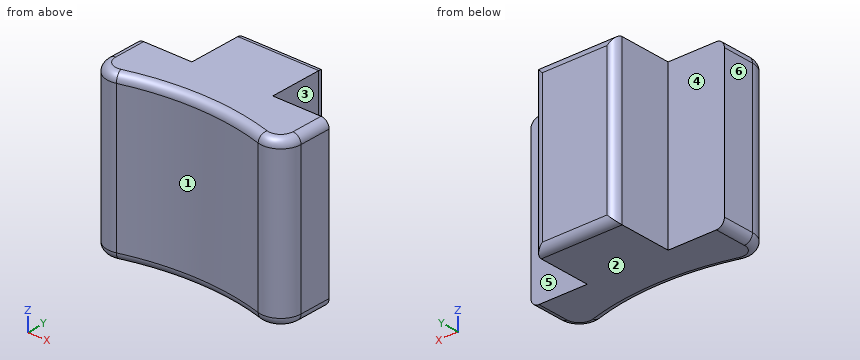
from build123d import *

# Parameters (mm, degrees)
BOSS_EXTRUDE1_DEPTH = 50.8
FILLET1_R           = 6.35
FILLET3_R           = 2.54
FILLET4_R           = 2.54
FILLET5_R           = 2.54


with BuildPart() as part:
    # Sketch1 → Boss-Extrude1 (new body)
    with BuildSketch(Plane.XY):
        with BuildLine():
            Line((-12.7, 111.432937893), (12.7, 111.432937893))
            Line((12.7, 111.432937893), (12.7, 92.382937893))
            Line((12.7, 92.382937893), (30.375497444, 92.382937893))
            Line((30.375497444, 92.382937893), (30.375497444, 73.332937893))
            ThreePointArc((30.375497444, 73.332937893), (0, 79.375), (-30.375497444, 73.332937893))
            Line((-30.375497444, 73.332937893), (-30.375497444, 92.382937893))
            Line((-30.375497444, 92.382937893), (-12.7, 92.382937893))
            Line((-12.7, 92.382937893), (-12.7, 111.432937893))
        make_face()
    extrude(amount=BOSS_EXTRUDE1_DEPTH)

    # Fillet1
    fillet1_edges = [part.edges().sort_by_distance(p)[0] for p in [
        (30.375497444, 73.332937893, 25.4),
        (-30.375497444, 73.332937893, 25.4),
    ]]
    fillet(fillet1_edges, radius=FILLET1_R)

    # Fillet3
    fillet3_edges = [part.edges().sort_by_distance(p)[0] for p in [
        (-12.7, 111.432937893, 25.4),
        (12.7, 111.432937893, 25.4),
        (0, 111.432937893, 50.8),
        (0, 111.432937893, 0),
    ]]
    fillet(fillet3_edges, radius=FILLET3_R)

    # Fillet4
    fillet4_edges = [part.edges().sort_by_distance(p)[0] for p in [
        (0, 79.375, 50.8),
        (30.375497444, 87.336186401, 50.8),
        (27.834803015, 77.208914161, 50.8),
        (-27.834803015, 77.208914161, 50.8),
        (-30.375497444, 87.336186401, 50.8),
    ]]
    fillet(fillet4_edges, radius=FILLET4_R)

    # Fillet5
    fillet5_edges = [part.edges().sort_by_distance(p)[0] for p in [
        (-30.375497444, 87.336186401, 0),
        (0, 79.375, 0),
        (30.375497444, 87.336186401, 0),
        (27.834803015, 77.208914161, 0),
        (-27.834803015, 77.208914161, 0),
    ]]
    fillet(fillet5_edges, radius=FILLET5_R)


solid = part.part
Work out the finished part from the listing and answer in its coordinate system (mm). Face numbers are marked on the shaded views. A direction names the side the tool comes from. Coordinates: 2 decimals unless noted, no trailing zeros. Loops run counter-clockwise (first coordinate to the right, second up) from the corner with the lowest first, then second, coordinate; pieces in that order, holes last. Notation, with made-up numbers: M -35,38.25 L -13,38.25 A22 ccw -13,75.25 Z; hole C -12,25 d1. An arc over 180 degrees is marked long. Answer in a Markdown table with one row per item. Add a question column.
1. Flat-ended cylindrical pins translate along their axes: P1, Ø12, axis at x = 4.5, y = 101.5, coming from the -Z side; P2, Ø2, axis at y = 106.5, z = 33.5, coming from the +X side; P3, Ø5.5, axis at x = 23.5, z = 19.5, coming from the +Y side; P4, Ø5, axis at y = 99, z = 13.5, coming from the -X side. Find the tip coordinate at first contact, or state that the pin passes through.
2. Find section B-B, the plane x = 0. Write down the section's boundary in (y, z) (3 decimals), then the cut area to 3 significant figures.
3. A tool of negligible diameter and unlimited length cuts with its end or side. For the marked faces 4, 5 and 6, from which of +Z, -Z, +X, -X, +Y, -Y can it reach the whole face along a straight path? Write none if from no direction.
4. The mould has two halves that part along X. Classify the marked faces 1, 2 and 3: pulls with the +X half, pulls with the -X half, needs draft (parallel to the pull), parting line crosses it, or undercut.
5. Consider L1, parallel to X at y = 108, z = 38; L2, parallel to X at y = 85, z = 48.5; L3, parallel to Y at x = -24, z = 44. Determine where each line is inside the solid, lowest interval first.
6. Find section C-C, the plane y = 101. Write down the section's boundary in (x, z), then the cut area to 3 significant figures.
Reported:
| question | item | result |
|---|---|---|
| 1 | P1 | stops at z = 0 |
| 1 | P2 | stops at x = 12.7 |
| 1 | P3 | stops at y = 92.38 |
| 1 | P4 | stops at x = -12.7 |
| 2 | outline | M 79.375,2.54 A2.54 ccw 81.915,0 L 108.893,0 A2.54 ccw 111.433,2.54 L 111.433,48.26 A2.54 ccw 108.893,50.8 L 81.915,50.8 A2.54 ccw 79.375,48.26 Z |
| 2 | area | 1,620 mm^2 |
| 3 | face 4 | +Z, -Z, -X, +Y |
| 3 | face 5 | +Z, -Z, +X, +Y |
| 3 | face 6 | +Z, -Z, -X, +Y, -Y |
| 4 | face 1 | undercut |
| 4 | face 2 | needs draft |
| 4 | face 3 | pulls with the +X half |
| 5 | L1 | x = -12.7 to 12.7 |
| 5 | L2 | x = -30.36 to 30.36 |
| 5 | L3 | y = 75.94 to 92.38 |
| 6 | outline | M -12.7,0 L 12.7,0 L 12.7,50.8 L -12.7,50.8 Z |
| 6 | area | 1,290 mm^2 |
